Drawing for the job (mm, zero at the part's lowest x, y, z). Give positions to 0.01 mm unless a question says otherwise; leave off trailing zeros. Order: outer loops, then holes, each group sorted by start corner. A loop starts at its lowest first (then second) coordinate and runs counter-clockwise, first axis right, second up. Notation, with made-up numbers: (-40, -32) -> (2, -32) arc R17 cw to (2, -26) -> close; hole circle Ø5 at (-13.5, -38). An arc over 180 degrees is marked (long way). Use one line per item in the form item = value. Start each with the question number.
1) Probe line 1 (Z direction, x = 41.5, y = 2.05); line 2 (X direction, y = 0.65, z = 26). List the from-to ranges inside material, lowest first.
2) Cut at A-A, the plane z = 26. Give the cut face in (x, y).
3) Cut at B-B, the plane x = 26. Give the cut face in (y, z).
4) Cut at C-C, the plane y = 2.15. Give the cut face in (x, z), and give its area (3 significant figures).
5) Drop flat-ended pins along their axis: P1, Ø2.5, axis at x = 41.5, z = 41.5, coming from the -Y side (3 decimals); P2, Ø5, axis at x = 41.5, z = 10.5, coming from the +Y side; P3, Ø1.5, axis at y = 1.5, z = 16.5, coming from the -X side. Give the stop position or say it passes through.
6) Cut at D-D, the plane x = 41.5. Give the cut face in (y, z).
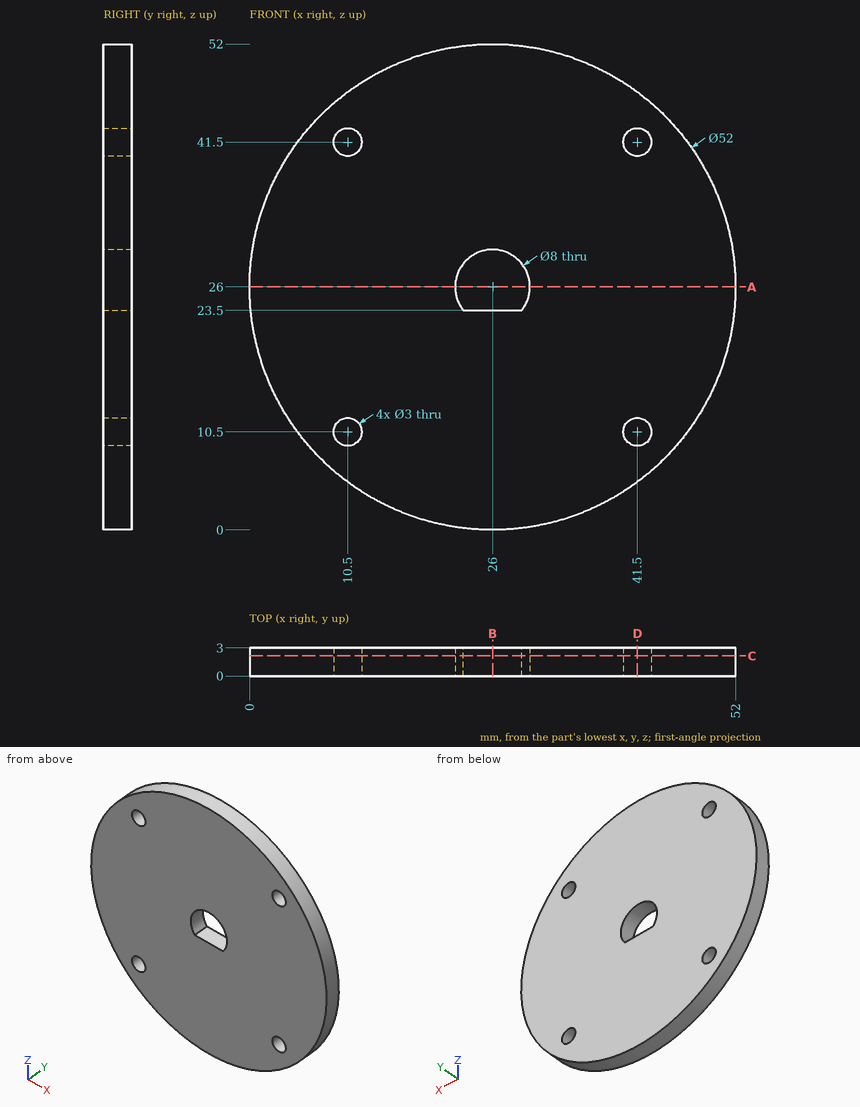
Result:
q1.line_1 = 5.13 to 9, 12 to 40, 43 to 46.87
q1.line_2 = 0 to 22, 30 to 52
q2.outline = (0, 0) -> (22, 0) -> (22, 3) -> (0, 3) -> close; (30, 0) -> (52, 0) -> (52, 3) -> (30, 3) -> close
q3.outline = (0, 0) -> (3, 0) -> (3, 23.5) -> (0, 23.5) -> close; (0, 30) -> (3, 30) -> (3, 52) -> (0, 52) -> close
q4.outline = circle Ø52 at (26, 26); hole circle Ø3 at (10.5, 10.5); hole circle Ø3 at (10.5, 41.5); hole (22.88, 23.5) -> (29.12, 23.5) arc R4 ccw (long way) to start; hole circle Ø3 at (41.5, 10.5); hole circle Ø3 at (41.5, 41.5)
q4.area = 2,050 mm²
q5.P1 = through
q5.P2 = 3
q5.P3 = 1.52
q6.outline = (0, 5.13) -> (3, 5.13) -> (3, 9) -> (0, 9) -> close; (0, 12) -> (3, 12) -> (3, 40) -> (0, 40) -> close; (0, 43) -> (3, 43) -> (3, 46.87) -> (0, 46.87) -> close
